from build123d import *

# Parameters (mm, degrees)
SKETCH_1_W            = 60
SKETCH_1_H            = 40
EXTRUDE_1_DEPTH       = 40
HOLE_WIZARD_5_DEPTH   = 40
HOLE_START            = 34.3
HOLE_WIZARD_5_2_DEPTH = 5.7
SKETCH_9_W            = 26
SKETCH_9_H            = 20
CUT_EXTRUDE_1_DEPTH   = 65.031242374
CHAMFER_1_SIZE        = 1


# Read off the part's stored shape, not the designer's step: 打孔尺寸(%根据)内六角圆柱头螺钉的类型5
with BuildPart() as part:
    # 草图1 → 凸台-拉伸1 (new body)
    with BuildSketch(Plane.XY):
        Rectangle(SKETCH_1_W, SKETCH_1_H)
    extrude(amount=EXTRUDE_1_DEPTH)

    # 打孔尺寸(%根据)内六角圆柱头螺钉的类型5 outline → 打孔尺寸(%根据)内六角圆柱头螺钉的类型5 (cut)
    with BuildSketch(Plane.XY):
        with BuildLine():
            Line((17.25, 4.75), (17.25, -4.75))
            ThreePointArc((17.25, -4.75), (20, -7.5), (22.75, -4.75))
            Line((22.75, -4.75), (22.75, 4.75))
            ThreePointArc((22.75, 4.75), (20, 7.5), (17.25, 4.75))
        make_face()
        with BuildLine():
            Line((-22.75, 4.75), (-22.75, -4.75))
            ThreePointArc((-22.75, -4.75), (-20, -7.5), (-17.25, -4.75))
            Line((-17.25, -4.75), (-17.25, 4.75))
            ThreePointArc((-17.25, 4.75), (-20, 7.5), (-22.75, 4.75))
        make_face()
    extrude(amount=HOLE_WIZARD_5_DEPTH, mode=Mode.SUBTRACT)

    # Hole Wizard 5 2 outline → Hole Wizard 5 2 (cut)
    # profile 1 of 2: a face of its own
    with BuildSketch(Plane.XY.offset(HOLE_START)):
        with BuildLine():
            Line((15, 4.75), (15, -4.75))
            ThreePointArc((15, -4.75), (20, -9.75), (25, -4.75))
            Line((25, -4.75), (25, 4.75))
            ThreePointArc((25, 4.75), (20, 9.75), (15, 4.75))
        make_face()
        with BuildLine():
            ThreePointArc((22.75, -4.75), (20, -7.5), (17.25, -4.75))
            Line((17.25, -4.75), (17.25, 4.75))
            ThreePointArc((17.25, 4.75), (20, 7.5), (22.75, 4.75))
            Line((22.75, 4.75), (22.75, -4.75))
        make_face(mode=Mode.SUBTRACT)
    # profile 2 of 2: a face of its own
    with BuildSketch(Plane.XY.offset(HOLE_START)):
        with BuildLine():
            Line((-25, 4.75), (-25, -4.75))
            ThreePointArc((-25, -4.75), (-20, -9.75), (-15, -4.75))
            Line((-15, -4.75), (-15, 4.75))
            ThreePointArc((-15, 4.75), (-20, 9.75), (-25, 4.75))
        make_face()
        with BuildLine():
            ThreePointArc((-17.25, -4.75), (-20, -7.5), (-22.75, -4.75))
            Line((-22.75, -4.75), (-22.75, 4.75))
            ThreePointArc((-22.75, 4.75), (-20, 7.5), (-17.25, 4.75))
            Line((-17.25, 4.75), (-17.25, -4.75))
        make_face(mode=Mode.SUBTRACT)
    extrude(amount=HOLE_WIZARD_5_2_DEPTH, mode=Mode.SUBTRACT)

    # 草图9 → 切除-拉伸1 (cut, through all)
    with BuildSketch(Plane.XZ.offset(20)):
        with Locations((0, 10)):
            Rectangle(SKETCH_9_W, SKETCH_9_H)
    extrude(amount=-CUT_EXTRUDE_1_DEPTH, mode=Mode.SUBTRACT)

    # 倒角1
    chamfer_1_edges = [part.edges().sort_by_distance(p)[0] for p in [
        (-30, 0, 40),
        (0, -20, 40),
        (30, 0, 40),
        (-21.5, -20, 0),
        (-30, 0, 0),
        (21.5, 20, 0),
        (21.5, -20, 0),
        (-21.5, 20, 0),
        (30, 0, 0),
        (13, 20, 10),
        (-13, 20, 10),
        (0, 20, 20),
        (13, -20, 10),
        (0, -20, 20),
        (-13, -20, 10),
        (0, 20, 40),
        (30, -20, 20),
        (-30, -20, 20),
        (-30, 20, 20),
        (30, 20, 20),
    ]]
    chamfer(chamfer_1_edges, length=CHAMFER_1_SIZE)


solid = part.part
Geometry: final body of the model. Coordinates: model frame, mm. A direction names the side the tool comes from. Give positions to 0.01 mm unless a question says otherwise; leave off trailing zeros. Write each loop counter-clockwise with the first axis right and the second up, starting at its lowest first coordinate (ties: lowest second). Pieces come first, ordered by that corner, then holes.
(1) Cut plane B-B, the plane z = 13. Return loops of the section in (x, y).
(2) Ray query, line 1 (X direction, y = -1.5, z = 30); line 2 (X direction, y = 4.5, z = 10); line 3 (X direction, y = 6, z = 29.5). Return the intervals inside material, ascending.
(3) Cut plane D-D, the plane z = 24.5. Return loops of the section in (x, y), then the cut area to 3 significant figures.
(4) Cut plane A-A, the plane y = -3.5. Return loops of the section in (x, z), then the cut area to 3 significant figures.
(5) Cut plane C-C, the plane x = 20. Return loops of the section in (y, z).
(6) Access query for faces 1 (the cylindrical face through (-20.1, -7.5, 16.9)), 2 (the flat face through (24, 0, 0)), 3 (the flat face through (13, 0, 10)), 4 (the flat face through (0, 20, 24)), 5 (the flat face through (-15, 0, 37)). Directions: +Z, -Z, +X, -X, +Y, -Y. A direction counts if a zero-diameter tool reaches every point of the face in a straight line with its end or side. Return the directions, or none.
(7) Mould query, pull axis X, two halves, no side actions, for faces 6 (the cylindrical face through (19.9, -7.5, 16.9)), 7 (the flat face through (-17, 0, 34.3)), 8 (the flat face through (0, -20, 24)), 9 (the flat face through (30, 0, 20)). Classes: released by +X, released by -X, zero draft, split by the parting line, or undercut.
Values follow:
1. outline: (-30, -19) - (-29, -20) - (-14, -20) - (-13, -19) - (-13, 19) - (-14, 20) - (-29, 20) - (-30, 19) - close; (13, -19) - (14, -20) - (29, -20) - (30, -19) - (30, 19) - (29, 20) - (14, 20) - (13, 19) - close; hole (-22.75, -4.75) arc R2.75 ccw to (-17.25, -4.75) - (-17.25, 4.75) arc R2.75 ccw to (-22.75, 4.75) - close; hole (17.25, -4.75) arc R2.75 ccw to (22.75, -4.75) - (22.75, 4.75) arc R2.75 ccw to (17.25, 4.75) - close
2. line 1: x = -30 to -22.75, -17.25 to 17.25, 22.75 to 30
2. line 2: x = -30 to -22.75, -17.25 to -13, 13 to 17.25, 22.75 to 30
2. line 3: x = -30 to -22.45, -17.55 to 17.55, 22.45 to 30
3. outline: (-30, -19) - (-29, -20) - (29, -20) - (30, -19) - (30, 19) - (29, 20) - (-29, 20) - (-30, 19) - close; hole (-22.75, -4.75) arc R2.75 ccw to (-17.25, -4.75) - (-17.25, 4.75) arc R2.75 ccw to (-22.75, 4.75) - close; hole (17.25, -4.75) arc R2.75 ccw to (22.75, -4.75) - (22.75, 4.75) arc R2.75 ccw to (17.25, 4.75) - close
3. area: 2,250 mm2
4. outline: (-30, 1) - (-29, 0) - (-22.75, 0) - (-22.75, 34.3) - (-25, 34.3) - (-25, 40) - (-29, 40) - (-30, 39) - close; (-17.25, 0) - (-13, 0) - (-13, 20) - (13, 20) - (13, 0) - (17.25, 0) - (17.25, 34.3) - (15, 34.3) - (15, 40) - (-15, 40) - (-15, 34.3) - (-17.25, 34.3) - close; (22.75, 0) - (29, 0) - (30, 1) - (30, 39) - (29, 40) - (25, 40) - (25, 34.3) - (22.75, 34.3) - close
4. area: 1,390 mm2
5. outline: (-20, 1) - (-19, 0) - (-7.5, 0) - (-7.5, 34.3) - (-9.75, 34.3) - (-9.75, 40) - (-19, 40) - (-20, 39) - close; (7.5, 0) - (19, 0) - (20, 1) - (20, 39) - (19, 40) - (9.75, 40) - (9.75, 34.3) - (7.5, 34.3) - close
6. face 1: +Z, -Z
6. face 2: -Z, +X, -X, +Y, -Y
6. face 3: -Z, +Y, -Y
6. face 4: +Z, -Z, +X, -X, +Y
6. face 5: +Z
7. face 6: undercut
7. face 7: undercut
7. face 8: zero draft
7. face 9: released by +X
